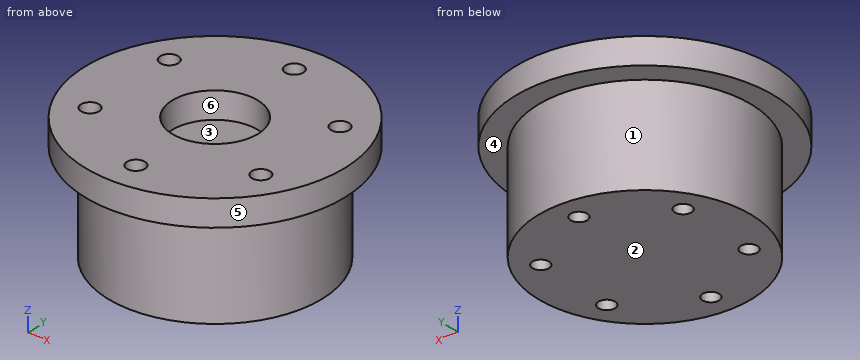
```python
from build123d import *

# Parameters (mm, degrees)
SKETCH1_R           = 39.5
SKETCH1_R_2         = 13.05
BOSS_EXTRUDE1_DEPTH = 8
SKETCH2_R           = 32.575
SKETCH2_R_2         = 2.55
BOSS_EXTRUDE3_DEPTH = 30
SKETCH1_5_R         = 2.75
CUT_EXTRUDE1_DEPTH  = 7


with BuildPart() as part:
    # Sketch1 → Boss-Extrude1 (new body)
    with BuildSketch(Plane.XY):
        Circle(SKETCH1_R)
        Circle(SKETCH1_R_2, mode=Mode.SUBTRACT)
    extrude(amount=-BOSS_EXTRUDE1_DEPTH)

    # Sketch2 → Boss-Extrude3 (add)
    with BuildSketch(Plane(origin=(0, 0, -8), x_dir=(-1, 0, 0), z_dir=(0, 0, -1))):
        Circle(SKETCH2_R)
        with Locations((0, 25)):
            Circle(SKETCH2_R_2, mode=Mode.SUBTRACT)
        with Locations((21.650635095, 12.5)):
            Circle(SKETCH2_R_2, mode=Mode.SUBTRACT)
        with Locations((21.650635095, -12.5)):
            Circle(SKETCH2_R_2, mode=Mode.SUBTRACT)
        with Locations((0, -25)):
            Circle(SKETCH2_R_2, mode=Mode.SUBTRACT)
        with Locations((-21.650635095, -12.5)):
            Circle(SKETCH2_R_2, mode=Mode.SUBTRACT)
        with Locations((-21.650635095, 12.5)):
            Circle(SKETCH2_R_2, mode=Mode.SUBTRACT)
    extrude(amount=BOSS_EXTRUDE3_DEPTH)

    # Sketch1_5 → Cut-Extrude1 (cut)
    with BuildSketch(Plane.XY):
        with Locations((-25.980762114, 15)):
            Circle(SKETCH1_5_R)
        with Locations((25.980762114, 15)):
            Circle(SKETCH1_5_R)
        with Locations((25.980762114, -15)):
            Circle(SKETCH1_5_R)
        with Locations((0, -30)):
            Circle(SKETCH1_5_R)
        with Locations((-25.980762114, -15)):
            Circle(SKETCH1_5_R)
        with Locations((0, 30)):
            Circle(SKETCH1_5_R)
    extrude(amount=-CUT_EXTRUDE1_DEPTH, mode=Mode.SUBTRACT)


solid = part.part
```
Read the model definition and answer for the solid it produces. Units are mm, in the model's axes. Face numbers are marked on the shaded views. A direction names the side the tool comes from. Round coordinates to 2 decimals unless told otherwise and drop trailing zeros. Write each loop counter-clockwise with the first axis right and the second up, starting at its lowest first coordinate (ties: lowest second). Pieces come first, ordered by that corner, then holes. Notation, with made-up numbers: (-6.75, -2.5) - (12.25, -2.5) arc R27 cw to (12.25, 22.5) - close; hole circle Ø10 at (86, -26). An arc over 180 degrees is marked (long way). Use CSV: the item, a comma, the result in double quotes.
Q1. Each of these flat-tipped pins is pushed along its axis until it touches: pin 1 Ø12 at (x, z) = (7.5, -10.5) entering from +Y; pin 2 Ø10 at (y, z) = (2, -19) entering from -X (3 decimals); pin 3 Ø10 at (x, z) = (-29.5, -26.5) entering from -Y. Where does it stop, or does it pass through?
Values:
pin 1,"stops at y = 39.45"
pin 2,"stops at x = -32.575"
pin 3,"stops at y = -21.47"
Q2. Straight lines are drawn through the part: line 1 along Y through (x, z) = (0, -3.25); line 2 along Y through (x, z) = (0, -14.75) (3 decimals); line 3 along Y through (x, z) = (-25, -4). For each, find the intervals that lie inside material, in ascending order.
Values:
line 1,"y = -39.5 to -32.75, -27.25 to -13.05, 13.05 to 27.25, 32.75 to 39.5"
line 2,"y = -32.575 to -27.55, -22.45 to 22.45, 27.55 to 32.575"
line 3,"y = -30.58 to -17.57, -12.43 to 12.43, 17.57 to 30.58"
Q3. Find section D-D, the plane y = -20.5. Write down the section's boundary in (x, z), then the cut area to 3 significant figures.
Values:
outline,"(-33.76, -8) - (-25.32, -8) - (-25.32, -38) - (25.32, -38) - (25.32, -8) - (33.76, -8) - (33.76, 0) - (-33.76, 0) - close"
area,"2,060 mm²"
Q4. Find section A-A, the plane z = -17.5. Write down the section's boundary in (x, y) (3 decimals).
Values:
outline,"circle Ø65.15 at (0, 0); hole circle Ø5.1 at (-21.651, -12.5); hole circle Ø5.1 at (-21.651, 12.5); hole circle Ø5.1 at (0, -25); hole circle Ø5.1 at (0, 25); hole circle Ø5.1 at (21.651, -12.5); hole circle Ø5.1 at (21.651, 12.5)"
Q5. A tool of negligible diameter and unlimited length cuts with its end or side. For the marked faces 4, 5 and 6, from which of +Z, -Z, +X, -X, +Y, -Y can it reach the whole face along a straight path? Write none if from no direction.
Values:
face 4,"-Z"
face 5,"+Z, -Z"
face 6,"+Z"
Q6. Find section C-C, the plane x = 6.5. Write down the section's boundary in (y, z), then the cut area to 3 significant figures.
Values:
outline,"(-38.96, -8) - (-31.92, -8) - (-31.92, -38) - (31.92, -38) - (31.92, -8) - (38.96, -8) - (38.96, 0) - (11.32, 0) - (11.32, -8) - (-11.32, -8) - (-11.32, 0) - (-38.96, 0) - close"
area,"2,360 mm²"
Q7. Determine the mould class of the marked faces 1, 2 and 3 for opening direction Y: +Y half, -Y half, draft (parallel to the pull), parting line (faces both ways), or undercut.
Values:
face 1,"parting line"
face 2,"draft"
face 3,"undercut"
Q8. Find section B-B, the plane y = 0. Write down the section's boundary in (x, z) (3 decimals), then the cut area to 3 significant figures.
Values:
outline,"(-39.5, -8) - (-32.575, -8) - (-32.575, -38) - (32.575, -38) - (32.575, -8) - (39.5, -8) - (39.5, 0) - (13.05, 0) - (13.05, -8) - (-13.05, -8) - (-13.05, 0) - (-39.5, 0) - close"
area,"2,380 mm²"
